Answer from the drawing. Dimensions are ordinates in mm from the lowest x, y and z of the part. A direction names the side the tool comes from. Give positions to 0.01 mm unless a question says otherwise; leave off trailing zeros. Order: outer loops, then holes, each group sorted by start corner. A loop starts at its lowest first (then second) coordinate and runs counter-clockwise, first axis right, second up.
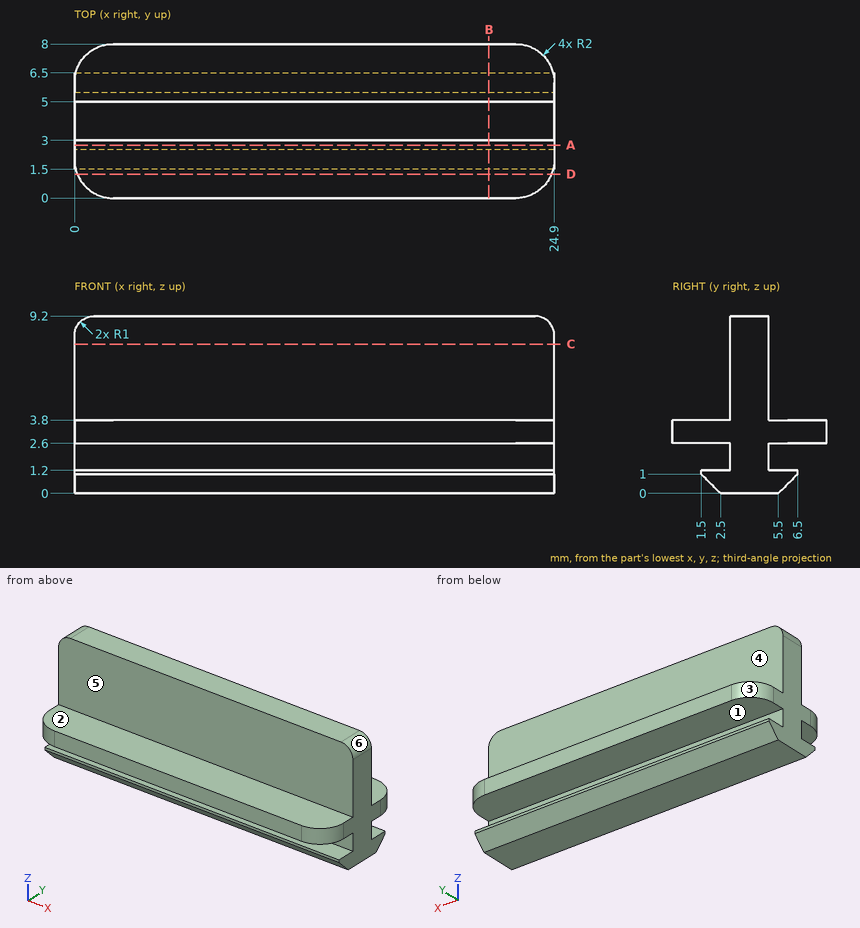
1. The part is cut by section A-A (y = 2.75). Write down the section's boundary in (x, z).
Findings below:
outline: (0, 0) - (24.9, 0) - (24.9, 1.2) - (0, 1.2) - close; (0, 2.6) - (24.9, 2.6) - (24.9, 3.8) - (0, 3.8) - close
2. Straight lines are drawn through the part: probe 1 along Y at (x, z) = (15, 7); probe 2 along Z at (x, y) = (19, 1.25); probe 3 along Z at (x, y) = (20.75, 1.75). For each, find the intervals that lie inside material, in ascending order.
Findings below:
probe 1: y = 3 to 5
probe 2: z = 2.6 to 3.8
probe 3: z = 0.75 to 1.2, 2.6 to 3.8
3. The part is cut by section C-C (z = 7.75). Write down the section's boundary in (x, y), then the cut area to 3 significant figures.
Findings below:
outline: (0, 3) - (24.9, 3) - (24.9, 5) - (0, 5) - close
area: 49.8 mm2
4. Given P1, Ø2.5, axis at x = 17, y = 1, coming from the +Z side; P2, Ø4.5, axis at x = 18, z = 7, coming from the +Y side; P3, Ø0.9, axis at x = 16.5, y = 2, coming from the -Z side, each flat-ended and moving along its own axis, determine where each tip first touches the part or whether it passes through.
Findings below:
P1: stops at z = 3.8
P2: stops at y = 5
P3: stops at z = 0.05
5. The part is cut by section D-D (y = 1.25). Write down the section's boundary in (x, z), then the cut area to 3 significant figures.
Findings below:
outline: (0.15, 2.6) - (24.75, 2.6) - (24.75, 3.8) - (0.15, 3.8) - close
area: 29.5 mm2
6. The part is cut by section B-B (x = 21.5). Write down the section's boundary in (y, z).
Findings below:
outline: (0, 2.6) - (3, 2.6) - (3, 1.2) - (1.5, 1.2) - (1.5, 1) - (2.5, 0) - (5.5, 0) - (6.5, 1) - (6.5, 1.2) - (5, 1.2) - (5, 2.6) - (8, 2.6) - (8, 3.8) - (5, 3.8) - (5, 9.2) - (3, 9.2) - (3, 3.8) - (0, 3.8) - close
7. The mould has two halves that part along Z. Classify the marked faces 1, 2 and 3: pulls with the +Z half, pulls with the -Z half, needs draft (parallel to the pull), parting line crosses it, or undercut.
Findings below:
face 1: undercut
face 2: pulls with the +Z half
face 3: needs draft
8. Which of the six approach directions +Z, -Z, +X, -X, +Y, -Y give full straight-line access (tool end or side, diameter ignored) to the marked faces 4, 5 and 6?
Findings below:
face 4: +Z, +X, -X, +Y
face 5: +Z, +X, -X, -Y
face 6: +Z, +X, +Y, -Y
